CAD build for the part. Positions are in the model's coordinates, mm. A direction names the side the tool comes from. Round coordinates to 2 decimals unless told otherwise and drop trailing zeros. Write each loop counter-clockwise with the first axis right and the second up, starting at its lowest first coordinate (ties: lowest second). Pieces come first, ordered by that corner, then holes. Notation, with made-up numbers: M -3.5,76.5 L 8.5,76.5 A31 ccw 8.5,111.5 Z; hole C 52.5,38.5 d10. An arc over 180 degrees is marked long. Write each question's results on one line, items separated by ' | '. Start each with the question number.
```python
from build123d import *

# Parameters (mm, degrees)
SKETCH1_R           = 51
BOSS_EXTRUDE1_DEPTH = 13
FILLET1_R           = 5
BOSS_EXTRUDE2_DEPTH = 13
SKETCH3_R           = 2.5
CUT_EXTRUDE1_DEPTH  = 13
SKETCH4_R           = 3
CUT_EXTRUDE2_DEPTH  = 16
SKETCH5_R           = 2.5
CUT_EXTRUDE3_DEPTH  = 132.918402101
FILLET2_R           = 3
CUT_EXTRUDE4_DEPTH  = 14
CUT_EXTRUDE5_DEPTH  = 14
FILLET3_R           = 3


with BuildPart() as part:
    # Sketch1 → Boss-Extrude1 (new body)
    with BuildSketch(Plane.XY):
        with BuildLine():
            Line((0, 0), (0, 200))
            Line((0, 200), (15, 200))
            Line((15, 200), (15, 180))
            Line((15, 180), (84.483320298, 161.323324697))
            ThreePointArc((84.483320298, 161.323324697), (131.5, 100), (84.483320298, 38.676675303))
            Line((84.483320298, 38.676675303), (15, 20))
            Line((15, 20), (15, 0))
            Line((15, 0), (0, 0))
        make_face()
        with Locations((68, 100)):
            Circle(SKETCH1_R, mode=Mode.SUBTRACT)
    extrude(amount=BOSS_EXTRUDE1_DEPTH)

    # Fillet1
    fillet1_edges = [part.edges().sort_by_distance(p)[0] for p in [
        (15, 180, 6.5),
        (15, 20, 6.5),
    ]]
    fillet(fillet1_edges, radius=FILLET1_R)

    # Sketch2 → Boss-Extrude2 (add)
    with BuildSketch(Plane.XY.offset(13)):
        with BuildLine():
            ThreePointArc((112.920417572, 144.882135479), (116.329690544, 141.188481545), (119.43612796, 137.236739123))
            Line((119.43612796, 137.236739123), (137.865467698, 150.141101731))
            Line((137.865467698, 150.141101731), (132.129703335, 158.332622174))
            Line((132.129703335, 158.332622174), (112.920417572, 144.882135479))
        make_face()
        with BuildLine():
            Line((139.012620571, 148.502797643), (120.583280833, 135.598435034))
            ThreePointArc((120.583280833, 135.598435034), (123.234239855, 131.327763208), (125.539099171, 126.860790505))
            Line((125.539099171, 126.860790505), (144.748384934, 140.3112772))
            Line((144.748384934, 140.3112772), (139.012620571, 148.502797643))
        make_face()
    extrude(amount=-BOSS_EXTRUDE2_DEPTH)

    # Sketch3 → Cut-Extrude1 (cut)
    with BuildSketch(Plane.XY.offset(13)):
        with Locations((96.625, 149.579954367)):
            Circle(SKETCH3_R)
        with Locations((124.38024386, 109.941358171)):
            Circle(SKETCH3_R)
        with Locations((87.580653205, 153.79740254)):
            Circle(SKETCH3_R)
        with Locations((77.941358171, 156.38024386)):
            Circle(SKETCH3_R)
        with Locations((68, 157.25)):
            Circle(SKETCH3_R)
        with Locations((58.058641829, 156.38024386)):
            Circle(SKETCH3_R)
        with Locations((48.419346795, 153.79740254)):
            Circle(SKETCH3_R)
        with Locations((39.375, 149.579954367)):
            Circle(SKETCH3_R)
        with Locations((31.200409345, 143.856044369)):
            Circle(SKETCH3_R)
        with Locations((24.143955631, 136.799590655)):
            Circle(SKETCH3_R)
        with Locations((18.420045633, 128.625)):
            Circle(SKETCH3_R)
        with Locations((14.20259746, 119.580653205)):
            Circle(SKETCH3_R)
        with Locations((11.61975614, 109.941358171)):
            Circle(SKETCH3_R)
        with Locations((10.75, 100)):
            Circle(SKETCH3_R)
        with Locations((11.61975614, 90.058641829)):
            Circle(SKETCH3_R)
        with Locations((14.20259746, 80.419346795)):
            Circle(SKETCH3_R)
        with Locations((18.420045633, 71.375)):
            Circle(SKETCH3_R)
        with Locations((24.143955631, 63.200409345)):
            Circle(SKETCH3_R)
        with Locations((31.200409345, 56.143955631)):
            Circle(SKETCH3_R)
        with Locations((39.375, 50.420045633)):
            Circle(SKETCH3_R)
        with Locations((48.419346795, 46.20259746)):
            Circle(SKETCH3_R)
        with Locations((58.058641829, 43.61975614)):
            Circle(SKETCH3_R)
        with Locations((68, 42.75)):
            Circle(SKETCH3_R)
        with Locations((77.941358171, 43.61975614)):
            Circle(SKETCH3_R)
        with Locations((87.580653205, 46.20259746)):
            Circle(SKETCH3_R)
        with Locations((96.625, 50.420045633)):
            Circle(SKETCH3_R)
        with Locations((104.799590655, 56.143955631)):
            Circle(SKETCH3_R)
        with Locations((111.856044369, 63.200409345)):
            Circle(SKETCH3_R)
        with Locations((117.579954367, 71.375)):
            Circle(SKETCH3_R)
        with Locations((121.79740254, 80.419346795)):
            Circle(SKETCH3_R)
        with Locations((124.38024386, 90.058641829)):
            Circle(SKETCH3_R)
        with Locations((125.25, 100)):
            Circle(SKETCH3_R)
    extrude(amount=-CUT_EXTRUDE1_DEPTH, mode=Mode.SUBTRACT)

    # Sketch4 → Cut-Extrude2 (cut, through all)
    with BuildSketch(Plane(origin=(15, 0, 0), x_dir=(0, 0, -1), z_dir=(1, 0, 0))):
        with Locations((-6.5, 191.916753533)):
            Circle(SKETCH4_R)
        with Locations((-6.5, 8.083246467)):
            Circle(SKETCH4_R)
    extrude(amount=-CUT_EXTRUDE2_DEPTH, mode=Mode.SUBTRACT)

    # Sketch5 → Cut-Extrude3 (cut, through all)
    with BuildSketch(Plane(origin=(-18.303975113, 26.140785572, 0), x_dir=(0.819152044, 0.573576436, 0), z_dir=(0.573576436, -0.819152044, 0))):
        with Locations((187.325073819, 6.5)):
            Circle(SKETCH5_R)
    extrude(amount=-CUT_EXTRUDE3_DEPTH, mode=Mode.SUBTRACT)

    # Fillet2
    fillet2_edges = [part.edges().sort_by_distance(p)[0] for p in [
        (112.920417572, 144.882135479, 6.5),
        (125.539099171, 126.860790505, 6.5),
    ]]
    fillet(fillet2_edges, radius=FILLET2_R)

    # Sketch6 → Cut-Extrude4 (cut, through all)
    with BuildSketch(Plane.XY.offset(13)):
        with BuildLine():
            Line((42.140126878, 162.34995559), (10, 170.989017617))
            Line((10, 170.989017617), (10, 134.528973341))
            ThreePointArc((10, 134.528973341), (23.822841385, 151.035562666), (42.140126878, 162.34995559))
        make_face()
    extrude(amount=-CUT_EXTRUDE4_DEPTH, mode=Mode.SUBTRACT)

    # Sketch7 → Cut-Extrude5 (cut, through all)
    with BuildSketch(Plane.XY.offset(13)):
        with BuildLine():
            Line((16.106302292, 30.652317666), (10, 29.010982383))
            Line((10, 29.010982383), (10, 65.471026659))
            ThreePointArc((10, 65.471026659), (23.822841385, 48.964437334), (42.140126878, 37.65004441))
            Line((42.140126878, 37.65004441), (16.106302292, 30.652317666))
        make_face()
    extrude(amount=-CUT_EXTRUDE5_DEPTH, mode=Mode.SUBTRACT)

    # Fillet3
    fillet3_edges = [part.edges().sort_by_distance(p)[0] for p in [
        (10, 134.528973341, 6.5),
        (10, 170.989017617, 6.5),
        (42.140126878, 162.34995559, 6.5),
        (10, 65.471026659, 6.5),
        (42.140126878, 37.65004441, 6.5),
        (10, 29.010982383, 6.5),
    ]]
    fillet(fillet3_edges, radius=FILLET3_R)


solid = part.part
```
1) Wall check: line 1 along Y through (x, z) = (3, 6.5); line 2 along Y through (x, z) = (105.5, 9); line 3 along Y through (x, z) = (60, 9). Give the ranges that are in metal, low to high. Write a range as from..to.
2) Drop flat-ended pins along their axis: pin 1 Ø5 at (x, z) = (20.5, 3.5) entering from -Y; pin 2 Ø5 at (x, z) = (34, 2) entering from +Y; pin 3 Ø3 at (y, z) = (69.5, 6.5) entering from +X. Give the stop position or say it passes through.
3) Saw through at A-A, the plane y = 100. Write the cut outline in (x, z), plus the area to 4 significant figures.
4) Saw through at B-B, the plane x = 68. Write the cut outline in (y, z), plus the area to 3 significant figures.
5) Pull direction Y, two halves, no side cores. Call faces 1 (the face through (0, 99, 6)), 2 (the face through (115.6, 69.85, 6.59)), 3 (the face through (7, 200, 6)), 4 (the face through (24.224, 167.166, 6.591)): pulls with the +Y half, pulls with the -Y half, needs draft (parallel to the pull), parting line crosses it, or undercut.
6) 3-axis set-ups, long thin cutter, end or side, ignore diameter. For faces 5 (the face through (11.96, 58.71, 6.41)), 6 (the face through (141.92, 144.35, 6.59)): which of +Z, -Z, +X, -X, +Y, -Y reach the whole face in a straight line?
Filled sheet:
1) line 1: y = 0..5.08, 11.08..188.92, 194.92..200 | line 2: y = 48.76..53.74, 58.54..65.43, 134.57..151.24 | line 3: y = 32.1..42.04, 45.19..49.63, 150.37..154.81, 157.96..167.9
2) pin 1: stops at y = 20.75 | pin 2: stops at y = 175.56 | pin 3: stops at x = 124.49
3) outline: M 0,0 L 8.25,0 L 8.25,13 L 0,13 Z; M 13.25,0 L 17,0 L 17,13 L 13.25,13 Z; M 119,0 L 122.75,0 L 122.75,13 L 119,13 Z; M 127.75,0 L 131.5,0 L 131.5,13 L 127.75,13 Z | area: 253.5 mm^2
4) outline: M 34.25,0 L 40.25,0 L 40.25,13 L 34.25,13 Z; M 45.25,0 L 49,0 L 49,13 L 45.25,13 Z; M 151,0 L 154.75,0 L 154.75,13 L 151,13 Z; M 159.75,0 L 165.75,0 L 165.75,13 L 159.75,13 Z | area: 254 mm^2
5) face 1: needs draft | face 2: undercut | face 3: pulls with the +Y half | face 4: undercut
6) face 5: +Z, -Z | face 6: +Z, -Z, +X, +Y
